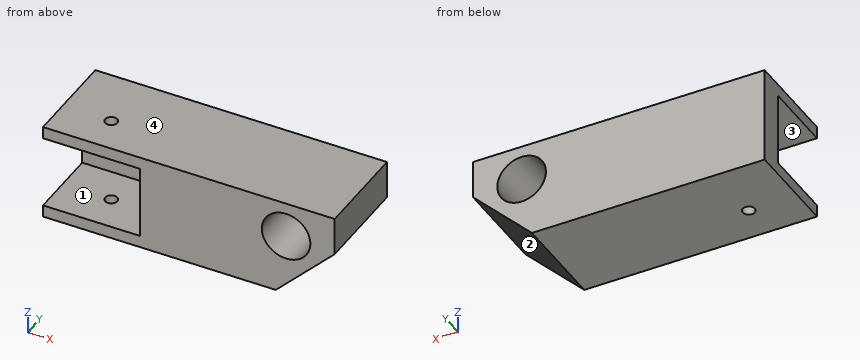
from build123d import *

# Parameters (mm, degrees)
F1_DEPTH = 50.8
F2_W     = 12.7
F2_H     = 38.1
F3_DEPTH = 50.8
F5_D     = 25.4
F7_D     = 6.35


# Not quite as in the source:
# - a feature names something its author has since deleted; it is built from what else it names


with BuildPart() as f1:
    # F0 (on Front) → F1 (new body)
    with BuildSketch(Plane.XZ):
        Polygon((-140.8084735786, 36.6746302678), (-140.8084735786, 30.3246302678), (-90.0084735786, 30.3246302678), (-90.0084735786, -7.7753697322), (-140.8084735786, -7.7753697322), (-140.8084735786, -14.1253697322), (-19.2084735786, -14.1253697322), (11.5915264214, 16.6746302678), (11.5915264214, 36.6746302678), align=None)
    extrude(amount=F1_DEPTH)

    # F2 (on face) → F3 (join)
    with BuildSketch(Plane(origin=(-90.0084735786, 0, 0), x_dir=(0, -1, 0), z_dir=(-1, 0, 0))):
        with Locations((6.35, 11.2746302678)):
            Rectangle(F2_W, F2_H)
    extrude(amount=F3_DEPTH)

    # F5 (through all)
    with Locations(Plane(origin=(0, 0, 0), x_dir=(-1, 0, 0), z_dir=(0, 1, 0))):
        with Locations((13.8084735786, 18.215398631)):
            Hole(F5_D / 2)

    # F7 (through all)
    with Locations(Plane.XY.offset(36.6746302678)):
        with Locations((-115.4084735786, -31.75)):
            Hole(F7_D / 2)


solid = f1.part
Can you work these out from the model? Positions are in its coordinate system, mm. Face numbers are marked on the shaded views. Round coordinates to 2 decimals unless told otherwise and drop trailing zeros. Loops run counter-clockwise (first coordinate to the right, second up) from the corner with the lowest first, then second, coordinate; pieces in that order, holes last. Notation, with made-up numbers: (-18.75, -19) - (-3.75, -19) arc R22 ccw to (-3.75, -9) - close; hole circle Ø4 at (-37, 3.5). An arc over 180 degrees is marked (long way). Write item = value, one per line. Start each with the question number.
(1) If we section it at C-C (x = -94): Please give me the cut outline in (y, z).
(2) If I drill on probe 1 along Z at (x, y) = (-131, -15); probe 2 along Y at (x, z) = (-115.5, -9); probe 3 along X at (y, z) = (-28.5, 24.5), over which ranges is the centre line in solid material (lowest first)? Write a range as [from, to].
(3) If we section it at D-D (y = -40): Please give me the cut outline in (x, z).
(4) If we section it at A-A (x = -15): Please give me the cut outline in (y, z), and give its area (3 significant figures).
(5) If we section it at B-B (y = -31.75): Please give me the cut outline in (x, z), and give its area (3 significant figures).
(6) For P1, Ø1, axis at x = -94.5, z = 20.5, coming from the -Y side; P2, Ø12, axis at y = -37, z = -1, coming from the -X side, each with a flat end and sliding along its axis, tell me the tip position at first contact or that it passes through.
(7) If we mould it in two halves opening along Z, with no side actions, what happens to the marked faces 1, 2, 3 and 4? For each: released by +Z, released by -Z, zero draft, split by the parting line, or undercut.
Ans:
q1.outline = (-50.8, -14.13) - (0, -14.13) - (0, 36.67) - (-50.8, 36.67) - (-50.8, 30.32) - (-12.7, 30.32) - (-12.7, -7.78) - (-50.8, -7.78) - close
q2.probe_1 = [-14.13, -7.78], [30.32, 36.67]
q2.probe_2 = [-50.8, -34.92], [-28.58, 0]
q2.probe_3 = [-90.01, -24.84], [-2.77, 11.59]
q3.outline = (-140.81, -14.13) - (-19.21, -14.13) - (11.59, 16.67) - (11.59, 36.67) - (-140.81, 36.67) - (-140.81, 30.32) - (-90.01, 30.32) - (-90.01, -7.78) - (-140.81, -7.78) - close; hole circle Ø25.4 at (-13.81, 18.22)
q4.outline = (-50.8, -9.92) - (0, -9.92) - (0, 5.57) - (-50.8, 5.57) - close; (-50.8, 30.86) - (0, 30.86) - (0, 36.67) - (-50.8, 36.67) - close
q4.area = 1,080 mm²
q5.outline = (-140.81, -14.13) - (-118.58, -14.13) - (-118.58, -7.78) - (-140.81, -7.78) - close; (-140.81, 30.32) - (-118.58, 30.32) - (-118.58, 36.67) - (-140.81, 36.67) - close; (-112.23, -14.13) - (-19.21, -14.13) - (11.59, 16.67) - (11.59, 36.67) - (-112.23, 36.67) - (-112.23, 30.32) - (-90.01, 30.32) - (-90.01, -7.78) - (-112.23, -7.78) - close; hole circle Ø25.4 at (-13.81, 18.22)
q5.area = 4,740 mm²
q6.P1 = -12.7
q6.P2 = -90.01
q7.face_1 = undercut
q7.face_2 = released by -Z
q7.face_3 = undercut
q7.face_4 = released by +Z
